Check sheet for the modelled part. Datum: model origin and axes. Units: mm. Face numbers are marked on the shaded views. A direction names the side the tool comes from. Round coordinates to 2 decimals unless told otherwise and drop trailing zeros. Order: outer loops, then holes, each group sorted by start corner. A loop starts at its lowest first (then second) coordinate and runs counter-clockwise, first axis right, second up. Notation, with made-up numbers: (48.5, 23) -> (52.5, 23) arc R24 cw to (52.5, 60) -> close; hole circle Ø10 at (-19, -23). An arc over 180 degrees is marked (long way). Use CSV: the item, a comma, the result in double quotes.
```python
from build123d import *

# Parameters (mm, degrees)
F1_DEPTH = 90.678


with BuildPart() as f1:
    # F0 (on Front) → F1 (new body)
    with BuildSketch(Plane.XZ):
        with BuildLine():
            Line((-38.8602614403, 7.4346788156), (-38.8602614403, 11.8796788156))
            Line((-38.8602614403, 11.8796788156), (-34.4152614403, 11.8796788156))
            ThreePointArc((-34.4152614403, 11.8796788156), (-42.0033510827, 15.022768458), (-38.8602614403, 7.4346788156))
        make_face()
        with BuildLine():
            Line((-34.4152614403, 11.8796788156), (-38.8602614403, 11.8796788156))
            Line((-38.8602614403, 11.8796788156), (-38.8602614403, 7.4346788156))
            ThreePointArc((-38.8602614403, 7.4346788156), (-35.7171717979, 8.7365891732), (-34.4152614403, 11.8796788156))
        make_face()
        with BuildLine():
            Line((34.4152614403, 11.8796788156), (-34.4152614403, 11.8796788156))
            ThreePointArc((-34.4152614403, 11.8796788156), (-35.7171717979, 8.7365891732), (-38.8602614403, 7.4346788156))
            Line((-38.8602614403, 7.4346788156), (-38.8602614403, -7.4346788156))
            ThreePointArc((-38.8602614403, -7.4346788156), (-35.7171717979, -8.7365891732), (-34.4152614403, -11.8796788156))
            Line((-34.4152614403, -11.8796788156), (34.4152614403, -11.8796788156))
            ThreePointArc((34.4152614403, -11.8796788156), (35.7171717979, -8.7365891732), (38.8602614403, -7.4346788156))
            Line((38.8602614403, -7.4346788156), (38.8602614403, 7.4346788156))
            ThreePointArc((38.8602614403, 7.4346788156), (35.7171717979, 8.7365891732), (34.4152614403, 11.8796788156))
        make_face()
        with BuildLine():
            ThreePointArc((43.3052614403, 11.8796788156), (38.8602614403, 16.3246788156), (34.4152614403, 11.8796788156))
            Line((34.4152614403, 11.8796788156), (38.8602614403, 11.8796788156))
            Line((38.8602614403, 11.8796788156), (38.8602614403, 7.4346788156))
            ThreePointArc((38.8602614403, 7.4346788156), (42.0033510827, 8.7365891732), (43.3052614403, 11.8796788156))
        make_face()
        with BuildLine():
            Line((38.8602614403, 11.8796788156), (34.4152614403, 11.8796788156))
            ThreePointArc((34.4152614403, 11.8796788156), (35.7171717979, 8.7365891732), (38.8602614403, 7.4346788156))
            Line((38.8602614403, 7.4346788156), (38.8602614403, 11.8796788156))
        make_face()
        with BuildLine():
            ThreePointArc((-34.4152614403, -11.8796788156), (-35.7171717979, -8.7365891732), (-38.8602614403, -7.4346788156))
            Line((-38.8602614403, -7.4346788156), (-38.8602614403, -11.8796788156))
            Line((-38.8602614403, -11.8796788156), (-34.4152614403, -11.8796788156))
        make_face()
        with BuildLine():
            Line((-38.8602614403, -11.8796788156), (-38.8602614403, -7.4346788156))
            ThreePointArc((-38.8602614403, -7.4346788156), (-42.0033510827, -15.022768458), (-34.4152614403, -11.8796788156))
            Line((-34.4152614403, -11.8796788156), (-38.8602614403, -11.8796788156))
        make_face()
        with BuildLine():
            ThreePointArc((43.3052614403, -11.8796788156), (42.0033510827, -8.7365891732), (38.8602614403, -7.4346788156))
            Line((38.8602614403, -7.4346788156), (38.8602614403, -11.8796788156))
            Line((38.8602614403, -11.8796788156), (34.4152614403, -11.8796788156))
            ThreePointArc((34.4152614403, -11.8796788156), (38.8602614403, -16.3246788156), (43.3052614403, -11.8796788156))
        make_face()
        with BuildLine():
            Line((38.8602614403, -11.8796788156), (38.8602614403, -7.4346788156))
            ThreePointArc((38.8602614403, -7.4346788156), (35.7171717979, -8.7365891732), (34.4152614403, -11.8796788156))
            Line((34.4152614403, -11.8796788156), (38.8602614403, -11.8796788156))
        make_face()
    extrude(amount=F1_DEPTH)


solid = f1.part
```
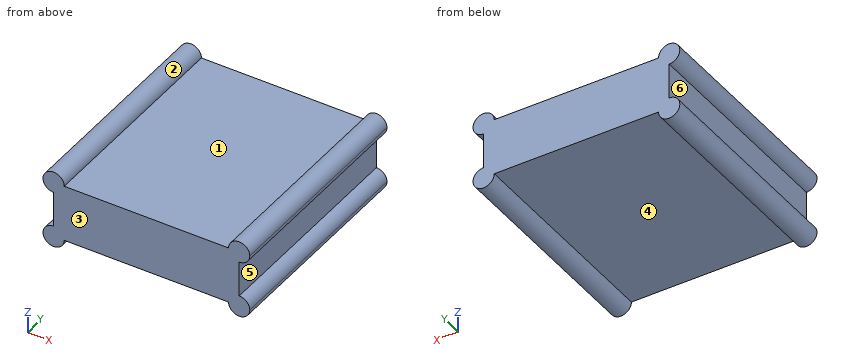
Q1. Scan lines: L1, parallel to X at y = -37, z = -7; L2, parallel to Z at x = -20.5, y = -43; L3, parallel to X at y = -15, z = 14. Record each from-to range of solid material in increasing order.
Result sheet:
L1,"x = -38.86 to 38.86"
L2,"z = -11.88 to 11.88"
L3,"x = -42.77 to -34.95, 34.95 to 42.77"
Q2. Mould release check, pull along Z, two halves, no side actions. Record for the marked faces 1, 2 and 3: pulls with the +Z half, pulls with the -Z half, needs draft (parallel to the pull), parting line crosses it, or undercut.
Result sheet:
face 1,"pulls with the +Z half"
face 2,"undercut"
face 3,"needs draft"
Q3. Sectioned sample at B-B, the plane y = -34. Enter the section's corners in (x, z) (3 decimals), then the cut area to 3 significant figures.
Result sheet:
outline,"(-38.86, -7.435) arc R4.445 ccw (long way) to (-34.415, -11.88) -> (34.415, -11.88) arc R4.445 ccw (long way) to (38.86, -7.435) -> (38.86, 7.435) arc R4.445 ccw (long way) to (34.415, 11.88) -> (-34.415, 11.88) arc R4.445 ccw (long way) to (-38.86, 7.435) -> close"
area,"2,030 mm^2"
Q4. Sectioned sample at D-D, the plane z = 5.5. Enter the section's corners in (x, y), then the cut area to 3 significant figures.
Result sheet:
outline,"(-38.86, -90.68) -> (38.86, -90.68) -> (38.86, 0) -> (-38.86, 0) -> close"
area,"7,050 mm^2"
Q5. Access from +Z, -Z, +X, -X, +Y, -Y to the whole of each face (thin tool, end or side, straight path). Record for the marked faces 4, 5 and 6.
Result sheet:
face 4,"-Z, +Y, -Y"
face 5,"+X, +Y, -Y"
face 6,"-X, +Y, -Y"
Q6. Sectioned sample at C-C, the plane x = 32.5. Enter the section's corners in (y, z).
Result sheet:
outline,"(-90.68, -11.88) -> (0, -11.88) -> (0, 11.88) -> (-90.68, 11.88) -> close"
Q7. Go/stop test with flat-tipped pins: pin 1 (4 mm diameter, centred on y = -23, z = 11, fed in from -X); pin 2 (20.5 mm diameter, centred on x = -7, y = -39.5, fed in from +Z); pin 3 (3 mm diameter, centred on y = -27.5, z = 3.5, fed in from -X); pin 4 (1 mm diameter, centred on y = -47.5, z = 5, fed in from +X). Record where each tip stops, or that it passes through.
Result sheet:
pin 1,"stops at x = -43.31"
pin 2,"stops at z = 11.88"
pin 3,"stops at x = -38.86"
pin 4,"stops at x = 38.86"
Q8. Sectioned sample at A-A, the plane z = -14. Enter the section's corners in (x, y).
Result sheet:
outline,"(-42.77, -90.68) -> (-34.95, -90.68) -> (-34.95, 0) -> (-42.77, 0) -> close; (34.95, -90.68) -> (42.77, -90.68) -> (42.77, 0) -> (34.95, 0) -> close"
